from build123d import *


with BuildPart() as part:
    # Sketch1 → Revolve1 (revolve)
    with BuildSketch(Plane.XY, mode=Mode.PRIVATE) as revolve1_sk:
        with BuildLine():
            Line((-0.85, 0), (-0.85, -1))
            Line((-0.85, -1), (-0.675, -1))
            Line((-0.675, -1), (-0.675, -4))
            Line((-0.675, -4), (-0.25, -4.736121593))
            Line((-0.25, -4.736121593), (-0.25, -8.8))
            ThreePointArc((-0.25, -8.8), (-0.176776695, -8.976776695), (0, -9.05))
            Line((0, -9.05), (0, 2.85))
            ThreePointArc((0, 2.85), (-0.176776695, 2.776776695), (-0.25, 2.6))
            Line((-0.25, 2.6), (-0.25, 0))
            Line((-0.25, 0), (-0.85, 0))
        make_face()
    revolve(revolve1_sk.sketch.rotate(Axis((0, 28.992562867, 0), (0, -1, 0)), 270), axis=Axis((0, 28.992562867, 0), (0, -1, 0)))


solid = part.part
Here's how the part is built. I have some questions about the finished solid (model axes, mm). A direction names the side the tool comes from. Coordinates: 2 decimals unless noted, no trailing zeros. Write each loop counter-clockwise with the first axis right and the second up, starting at its lowest first coordinate (ties: lowest second). Pieces come first, ordered by that corner, then holes.
Item 1: I want a section at A-A on z = 0. Write out the boundary of the cut face in (x, y) (3 decimals), and give its area (3 significant figures).
Item 2: I want a section at D-D on y = 0.25. Write out the boundary of the cut face in (x, z), and give its area (3 significant figures).
Item 3: I want a section at B-B on x = 0. Write out the boundary of the cut face in (y, z) (3 decimals).
Item 4: If I drill on line 1 (Y direction, x = -0.65, z = 0.45); line 2 (X direction, y = -3, z = 0.55); line 3 (Z direction, x = -0.2, y = -2.75), over which ranges is the centre line in solid material (lowest first)?
Item 5: On a 3-axis mill with a long thin cutter (end or side, diameter ignored), from which of +Z, -Z, +X, -X, +Y, -Y can I reach the whole of each face in a straight line? I mean faces 1 (the flat face through (0, 0, -0.4)), 2 (the cylindrical face through (-0.203, -2.521, 0.644)), 3 (the cylindrical face through (0.83, -0.51, -0.18)). Say none if no direction works.
Item 6: I want a section at C-C on y = -1.5. Write out the boundary of the cut face in (x, z) (3 decimals), and give its area (3 significant figures).
Item 7: Will these pins go through, and if not, where does the flat tip stop? pin 1 (0.8 mm diameter, centred on x = -0.5, z = 0.5, fed in from +Y); pin 2 (0.8 mm diameter, centred on x = 0.5, z = -0.5, fed in from -Y); pin 3 (1 mm diameter, centred on y = -5.5, z = 0.5, fed in from +X).
Findings below:
1. outline: (-0.85, -1) - (-0.675, -1) - (-0.675, -4) - (-0.25, -4.736) - (-0.25, -8.8) arc R0.25 ccw to (0.25, -8.8) - (0.25, -4.736) - (0.675, -4) - (0.675, -1) - (0.85, -1) - (0.85, 0) - (0.25, 0) - (0.25, 2.6) arc R0.25 ccw to (-0.25, 2.6) - (-0.25, 0) - (-0.85, 0) - close
1. area: 9.96 mm2
2. outline: circle Ø0.5 at (0, 0)
2. area: 0.196 mm2
3. outline: (-8.8, -0.25) - (-4.736, -0.25) - (-4, -0.675) - (-1, -0.675) - (-1, -0.85) - (0, -0.85) - (0, -0.25) - (2.6, -0.25) arc R0.25 ccw to (2.6, 0.25) - (0, 0.25) - (0, 0.85) - (-1, 0.85) - (-1, 0.675) - (-4, 0.675) - (-4.736, 0.25) - (-8.8, 0.25) arc R0.25 ccw to start
4. line 1: y = -1 to 0
4. line 2: x = -0.39 to 0.39
4. line 3: z = -0.64 to 0.64
5. face 1: +Y
5. face 2: -Y
5. face 3: +Y, -Y
6. outline: circle Ø1.35 at (0, 0)
6. area: 1.43 mm2
7. pin 1: stops at y = 0
7. pin 2: stops at y = -4.64
7. pin 3: stops at x = 0.25
